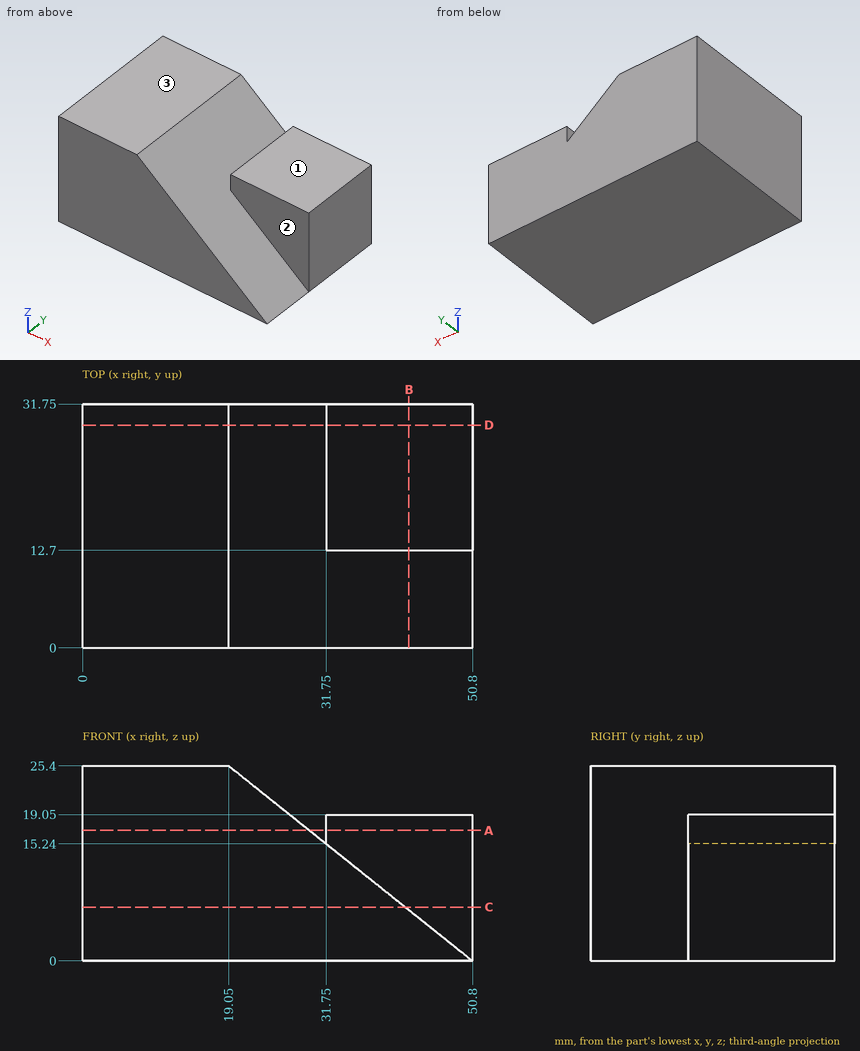
For this review, use the dimensioned drawing (mm, ordinates from the lowest corner) and the shaded views. A direction names the side the tool comes from. Coordinates: 2 decimals unless noted, no trailing zeros. Loops run counter-clockwise (first coordinate to the right, second up) from the corner with the lowest first, then second, coordinate; pieces in that order, holes last. Notation, with made-up numbers: (58.25, 59) -> (104.25, 59) arc R34 ccw to (104.25, 95) -> close; hole circle Ø10 at (14.5, -37.75). An arc over 180 degrees is marked (long way). Return JSON: item names as keys, results as strings. Group by question number.
(1) For pin 1 Ø5.5 at (x, z) = (45, 11.5) entering from -Y; pin 2 Ø1 at (y, z) = (10.5, 19.5) entering from +X; pin 3 Ø5 at (y, z) = (25.5, 10.5) entering from -X; pin 4 Ø6 at (x, y) = (34, 17.5) entering from +Z, all flat-tipped, find the tip position at first contact; note any pin that passes through.
(2) Consider section C-C, the plane z = 7. Give the boundary of the cut face in (x, y), plus the area to 3 significant figures.
(3) Consider section A-A, the plane z = 17. Give the boundary of the cut face in (x, y).
(4) Consider section D-D, the plane y = 29. Give the boundary of the cut face in (x, z).
(5) Tool access review of the marked faces 1, 2 and 3: name each direction out of +Z, -Z, +X, -X, +Y, -Y from which nothing blocks a thin tool from reaching the whole face with its end or side.
(6) Consider section B-B, the plane x = 42.5. Give the boundary of the cut face in (y, z), plus the area to 3 significant figures.
(7) To check wall thickness, follow L1, parallel to Z at x = 42, y = 20; L2, parallel to Y at x = 44.5, z = 11.75; L3, parallel to X at y = 10, z = 19. State the ranges of each line that lie inside material, in increasing order.
Results below:
{
 "1": {"pin 1": "stops at y = 12.7", "pin 2": "stops at x = 27.05", "pin 3": "stops at x = 0", "pin 4": "stops at z = 19.05"},
 "2": {"outline": "(0, 0) -> (42.05, 0) -> (42.05, 12.7) -> (50.8, 12.7) -> (50.8, 31.75) -> (0, 31.75) -> close", "area": "1,500 mm2"},
 "3": {"outline": "(0, 0) -> (29.55, 0) -> (29.55, 31.75) -> (0, 31.75) -> close; (31.75, 12.7) -> (50.8, 12.7) -> (50.8, 31.75) -> (31.75, 31.75) -> close"},
 "4": {"outline": "(0, 0) -> (50.8, 0) -> (50.8, 19.05) -> (31.75, 19.05) -> (31.75, 15.24) -> (19.05, 25.4) -> (0, 25.4) -> close"},
 "5": {"face 1": "+Z, +X, +Y, -Y", "face 2": "+Z, +X, -Y", "face 3": "+Z, +X, -X, +Y, -Y"},
 "6": {"outline": "(0, 0) -> (31.75, 0) -> (31.75, 19.05) -> (12.7, 19.05) -> (12.7, 6.64) -> (0, 6.64) -> close", "area": "447 mm2"},
 "7": {"L1": "z = 0 to 19.05", "L2": "y = 12.7 to 31.75", "L3": "x = 0 to 27.05"}
}
